The model under review builds one solid part; all positions refer to its coordinate system, in mm. A direction names the side the tool comes from. Coordinates: 2 decimals unless noted, no trailing zeros. Loops run counter-clockwise (first coordinate to the right, second up) from the corner with the lowest first, then second, coordinate; pieces in that order, holes last. Notation, with made-up numbers: M 51,22 L 73,22 A11 ccw 73,30 Z; hole C -16.75,82.5 d5. An arc over 180 degrees is marked long. Return JSON: item names as keys, results as strings.
```python
from build123d import *

# Parameters (mm, degrees)
BOSS_EXTRUDE1_DEPTH      = 20
BOSS_EXTRUDE1_DEPTH_BACK = 20
SKETCH1_W                = 134
SKETCH1_H                = 40
CUT_EXTRUDE1_DEPTH       = 40
FILLET1_R                = 20
FILLET2_R                = 4
SKETCH3_R                = 10
CUT_EXTRUDE2_DEPTH       = 29
SKETCH4_R                = 6
CUT_EXTRUDE3_DEPTH       = 11


with BuildPart() as part:
    # Sketch1 → Boss-Extrude1 (new, two sides: drawn at the far end of the back side and taken through both)
    with BuildSketch(Plane.XY.offset(-BOSS_EXTRUDE1_DEPTH_BACK)):
        Rectangle(SKETCH1_W, SKETCH1_H)
    extrude(amount=BOSS_EXTRUDE1_DEPTH + BOSS_EXTRUDE1_DEPTH_BACK)

    # Sketch2 → Cut-Extrude1 (cut)
    with BuildSketch(Plane.XY.offset(20)):
        Polygon((8, 20), (67, -1), (67, 20), align=None)
    extrude(amount=-CUT_EXTRUDE1_DEPTH, mode=Mode.SUBTRACT)

    # Fillet1
    fillet1_edges = [part.edges().sort_by_distance(p)[0] for p in [
        (8, 20, 0),
    ]]
    fillet(fillet1_edges, radius=FILLET1_R)

    # Fillet2
    fillet2_edges = [part.edges().sort_by_distance(p)[0] for p in [
        (67, -1, 0),
    ]]
    fillet(fillet2_edges, radius=FILLET2_R)

    # Sketch3 → Cut-Extrude2 (cut)
    with BuildSketch(Plane(origin=(0, 20, 0), x_dir=(1, 0, 0), z_dir=(0, 1, 0))):
        with Locations(Location((-47, 0, 0), (0, 0, 270))):
            Circle(SKETCH3_R)
        with Locations(Location((38, 0, 0), (0, 0, 270))):
            Circle(SKETCH3_R)
    extrude(amount=-CUT_EXTRUDE2_DEPTH, mode=Mode.SUBTRACT)

    # Sketch4 → Cut-Extrude3 (cut)
    with BuildSketch(Plane(origin=(0, -9, 0), x_dir=(1, 0, 0), z_dir=(0, 1, 0))):
        with Locations(Location((-47, 0, 0), (0, 0, 270))):
            Circle(SKETCH4_R)
        with Locations(Location((38, 0, 0), (0, 0, 270))):
            Circle(SKETCH4_R)
    extrude(amount=-CUT_EXTRUDE3_DEPTH, mode=Mode.SUBTRACT)


solid = part.part
```
1. Add section D-D on x = 56.5. Give the boundary of the cut face in (y, z).
Check values:
{"outline": "M -20,-20 L 2.74,-20 L 2.74,20 L -20,20 Z"}
2. The part is to be moulded in two halves that separate along Z. For faces 3 (the face through (31, -9, 0)), 4 (the face through (-1, 0, 20)), 5 (the face through (67, -12, 0)), 6 (the face through (32.143, -14.423, -1.301)), say which applies: released by +Z, released by -Z, zero draft, split by the parting line, or undercut.
Check values:
{"face 3": "undercut", "face 4": "released by +Z", "face 5": "zero draft", "face 6": "undercut"}
3. Machinability: for faces 1 (the face through (28.24, -0.34, -2.17)), 2 (the face through (7.902, 19.716, -0.28)), which of the approach directions +Z, -Z, +X, -X, +Y, -Y give a long, thin tool a straight path to every point of the face, cutting with its end or side? Answer none if there is none.
Check values:
{"face 1": "+Y", "face 2": "+Z, -Z, +X, +Y"}
4. Add section C-C on x = 34. Give the boundary of the cut face in (y, z).
Check values:
{"outline": "M -20,-20 L 10.75,-20 L 10.75,-9.17 L -9,-9.17 L -9,-4.47 L -20,-4.47 Z; M -20,4.47 L -9,4.47 L -9,9.17 L 10.75,9.17 L 10.75,20 L -20,20 Z"}
5. Insertion check: pin 1 Ø16 at (x, z) = (38, 0) entering from -Y; pin 2 Ø6 at (x, z) = (-47, 5) entering from +Y. Each pin has a flat end and moves straight along its axis. Give the tip position at first contact, or say it passes through.
Check values:
{"pin 1": "y = -20", "pin 2": "y = -9"}
6. Add section B-B on z = 0. Give the boundary of the cut face in (x, y).
Check values:
{"outline": "M -67,-20 L -53,-20 L -53,-9 L -57,-9 L -57,20 L -67,20 Z; M -41,-20 L 32,-20 L 32,-9 L 28,-9 L 28,12.88 L 11.25,18.84 A20 ccw 4.55,20 L -37,20 L -37,-9 L -41,-9 Z; M 44,-20 L 67,-20 L 67,-3.82 A4 ccw 64.34,-0.05 L 48,5.76 L 48,-9 L 44,-9 Z"}
7. Add section A-A on x = -47. Give the boundary of the cut face in (y, z).
Check values:
{"outline": "M -20,-20 L 20,-20 L 20,-10 L -9,-10 L -9,-6 L -20,-6 Z; M -20,6 L -9,6 L -9,10 L 20,10 L 20,20 L -20,20 Z"}
8. To check wall thickness, follow line 1 (X direction, y = -3.5, z = 0); line 2 (Z direction, x = 38, y = 4); line 3 (Y direction, x = 47.5, z = 2). State the ranges of each line that lie inside material, in increasing order.
Check values:
{"line 1": "-67 to -57, -37 to 28, 48 to 66.99", "line 2": "-20 to -10, 10 to 20", "line 3": "-20 to -9"}
